from build123d import *

# Parameters (mm, degrees)
SZKIC1_R                    = 3
DODANIE_WYCI_GNI_CIE1_DEPTH = 2
ZAOKR_GLENIE2_R             = 5


with BuildPart() as part:
    # Szkic1 → Dodanie-wyciągnięcie1 (new body)
    with BuildSketch(Plane.XY):
        Polygon((-6.588738933, 8), (6.588738933, 8), (23.822043257, 17), (31.525212111, 17), (36.579652034, 7.321699847), (32.177956743, 1), (14.944652418, -8), (-14.944652418, -8), (-32.177956743, 1), (-36.579652034, 7.321699847), (-31.525212111, 17), (-23.822043257, 17), align=None)
        Circle(SZKIC1_R, mode=Mode.SUBTRACT)
        with Locations((28, 9)):
            Circle(SZKIC1_R, mode=Mode.SUBTRACT)
        with Locations((-28, 9)):
            Circle(SZKIC1_R, mode=Mode.SUBTRACT)
    extrude(amount=DODANIE_WYCI_GNI_CIE1_DEPTH)

    # Zaokrąglenie2
    zaokr_glenie2_edges = [part.edges().sort_by_distance(p)[0] for p in [
        (6.588738933, 8, 1),
        (23.822043257, 17, 1),
        (31.525212111, 17, 1),
        (36.579652034, 7.321699847, 1),
        (32.177956743, 1, 1),
        (14.944652418, -8, 1),
        (-14.944652418, -8, 1),
        (-32.177956743, 1, 1),
        (-36.579652034, 7.321699847, 1),
        (-31.525212111, 17, 1),
        (-23.822043257, 17, 1),
        (-6.588738933, 8, 1),
    ]]
    fillet(zaokr_glenie2_edges, radius=ZAOKR_GLENIE2_R)


solid = part.part
Verification items for the finished model (mm, model axes). A direction names the side the tool comes from. Coordinates: 2 decimals unless noted, no trailing zeros. Order: outer loops, then holes, each group sorted by start corner. A loop starts at its lowest first (then second) coordinate and runs counter-clockwise, first axis right, second up. Notation, with made-up numbers: M -11.5,59.25 L 34.5,59.25 A33 cw 34.5,87.25 Z; hole C 87.25,21.5 d5. An arc over 180 degrees is marked long. Return JSON: item names as keys, results as strings.
1) Cross-section at C-C, the plane y = 7. Record the boundary of the cut face in (x, z).
Answer list:
{"outline": "M -35.7,0 L -30.24,0 L -30.24,2 L -35.7,2 Z; M -25.76,0 L 25.76,0 L 25.76,2 L -25.76,2 Z; M 30.24,0 L 35.7,0 L 35.7,2 L 30.24,2 Z"}
2) Access from +Z, -Z, +X, -X, +Y, -Y to the whole of each face (thin tool, end or side, straight path). Record for faces 4 (the flat face through (15.1, 12.445, 0.986)), 5 (the cylindrical face through (-31.05, 16.3, 1.01)).
Answer list:
{"face 4": "+Z, -Z, +Y", "face 5": "+Z, -Z, -X, +Y"}
3) Thickness scan on L1, parallel to X at y = 6.25, z = 1.6; L2, parallel to Y at x = 0, z = 1.2; L3, parallel to X at y = 15.5, z = 1.25. Record the ranges inside material, lowest first. Write a range as [from, to].
Answer list:
{"L1": "[-35.53, -29.2], [-26.8, 26.8], [29.2, 35.53]", "L2": "[-8, -3], [3, 8]", "L3": "[-32.07, -20.95], [20.95, 32.07]"}
4) Release check for a two-part mould opening along X. For faces 1 (the cylindrical face through (6.54, 8.14, 1.01)), 2 (the flat face through (33.878, 3.441, 0.986)), 3 (the flat face through (-23.456, -3.555, 0.986)) record: +X half, -X half, draft (parallel to the pull), parting line (faces both ways), or undercut.
Answer list:
{"face 1": "undercut", "face 2": "+X half", "face 3": "-X half"}
5) Cross-section at B-B, the plane z = 0.65. Record the boundary of the cut face in (x, y), and give its area (3 significant figures).
Answer list:
{"outline": "M -35.18,10.01 A5 ccw -34.85,4.84 L -32.88,2.01 A5 ccw -31.09,0.43 L -16.03,-7.43 A5 ccw -13.72,-8 L 13.72,-8 A5 ccw 16.03,-7.43 L 31.09,0.43 A5 ccw 32.88,2.01 L 34.85,4.84 A5 ccw 35.18,10.01 L 32.93,14.31 A5 ccw 28.5,17 L 25.05,17 A5 ccw 22.73,16.43 L 7.68,8.57 A5 cw 5.36,8 L -5.36,8 A5 cw -7.68,8.57 L -22.73,16.43 A5 ccw -25.05,17 L -28.5,17 A5 ccw -32.93,14.31 Z; hole C -28,9 d6; hole C 0,0 d6; hole C 28,9 d6", "area": "1,150 mm2"}
6) Cross-section at D-D, the plane y = -1.5. Record the boundary of the cut face in (x, z).
Answer list:
{"outline": "M -27.39,0 L -2.6,0 L -2.6,2 L -27.39,2 Z; M 2.6,0 L 27.39,0 L 27.39,2 L 2.6,2 Z"}
7) Cross-section at A-A, the plane y = 11. Record the boundary of the cut face in (x, z).
Answer list:
{"outline": "M -34.66,0 L -30.24,0 L -30.24,2 L -34.66,2 Z; M -25.76,0 L -12.33,0 L -12.33,2 L -25.76,2 Z; M 12.33,0 L 25.76,0 L 25.76,2 L 12.33,2 Z; M 30.24,0 L 34.66,0 L 34.66,2 L 30.24,2 Z"}
